```python
from build123d import *

# Parameters (mm, degrees)
F0_R     = 2
F1_DEPTH = 1


with BuildPart() as f1:
    # F0 (on Front) → F1 (new body)
    with BuildSketch(Plane.XZ):
        with BuildLine():
            Line((-30.187501, 20.062501), (-30.187501, -13.937499))
            Line((-30.187501, -13.937499), (-22.187501, -13.937499))
            ThreePointArc((-22.187501, -13.937499), (-17.94486, -12.18014), (-16.187501, -7.937499))
            Line((-16.187501, -7.937499), (-16.187501, 14.062501))
            ThreePointArc((-16.187501, 14.062501), (-17.94486, 18.305141), (-22.187501, 20.062501))
            Line((-22.187501, 20.062501), (-30.187501, 20.062501))
        make_face()
        with Locations((-23.125804, -9.637499)):
            Circle(F0_R, mode=Mode.SUBTRACT)
        with Locations((-23.125804, 2.785767)):
            Circle(F0_R, mode=Mode.SUBTRACT)
        with Locations((-23.125804, 15.079059)):
            Circle(F0_R, mode=Mode.SUBTRACT)
    extrude(amount=F1_DEPTH)


solid = f1.part
```
Geometry check sheet. Reference: the model listing, model coordinates, mm. Coordinates: 2 decimals unless noted, no trailing zeros. Order: outer loops, then holes, each group sorted by start corner. A loop starts at its lowest first (then second) coordinate and runs counter-clockwise, first axis right, second up.
Item 1: Scan lines: line 1 along Z through (x, y) = (-24.5, -0.85); line 2 along Z through (x, y) = (-22, -0.1); line 3 along X through (y, z) = (-0.5, 1.5). Record each from-to range of solid material in increasing order.
Item 2: Section check A-A (z = -9). Enter the section's corners in (x, y).
Item 3: Section check C-C (y = -0.3). Enter the section's corners in (x, z), plus the area to 3 significant figures.
Item 4: Section check D-D (z = 17.5). Enter the section's corners in (x, y).
Item 5: Mould release check, pull along X, two halves, no side actions. Record for faces 1 (the flat face through (-26, 0, 3)), 2 (the cylindrical face through (-25.124, -0.493, 2.874)), 3 (the cylindrical face through (-17.992, -0.493, -12.227)): released by +X, released by -X, zero draft, split by the parting line, or undercut.
Item 6: Section check B-B (x = -24). Enter the section's corners in (y, z).
Item 7: Depth check by flat-ended pin: pin 1 (6.5 mm diameter, centred on x = -23.13, z = 15.08, fed in from +Y). Enter the tip coordinate at first touch or a pass-through.
Check sheet entries:
1. line 1: z = -13.94 to -11.09, -8.18 to 1.33, 4.24 to 13.63, 16.53 to 20.06
1. line 2: z = -13.93 to -11.29, -7.98 to 1.13, 4.44 to 13.43, 16.73 to 20.06
1. line 3: x = -30.19 to -24.66, -21.59 to -16.19
2. outline: (-30.19, -1) - (-25.02, -1) - (-25.02, 0) - (-30.19, 0) - close; (-21.23, -1) - (-16.28, -1) - (-16.28, 0) - (-21.23, 0) - close
3. outline: (-30.19, -13.94) - (-22.19, -13.94) arc R6 ccw to (-16.19, -7.94) - (-16.19, 14.06) arc R6 ccw to (-22.19, 20.06) - (-30.19, 20.06) - close; hole circle Ø4 at (-23.13, -9.64); hole circle Ø4 at (-23.13, 2.79); hole circle Ø4 at (-23.13, 15.08)
3. area: 423 mm2
4. outline: (-30.19, -1) - (-17.27, -1) - (-17.27, 0) - (-30.19, 0) - close
5. face 1: zero draft
5. face 2: undercut
5. face 3: released by +X
6. outline: (-1, -13.94) - (0, -13.94) - (0, -11.44) - (-1, -11.44) - close; (-1, -7.84) - (0, -7.84) - (0, 0.99) - (-1, 0.99) - close; (-1, 4.58) - (0, 4.58) - (0, 13.28) - (-1, 13.28) - close; (-1, 16.88) - (0, 16.88) - (0, 20.06) - (-1, 20.06) - close
7. pin 1: stops at y = 0
